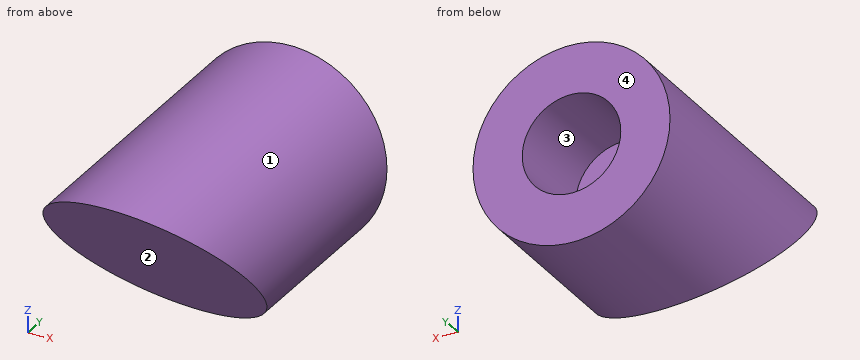
```python
from build123d import *

# Parameters (mm, degrees)
F0_R     = 5
F1_DEPTH = 12.5
F3_W     = 50
F3_H     = 50
F4_DEPTH = 25
F5_R     = 2.5
F6_DEPTH = 5


with BuildPart() as f1:
    # F0 (on Front) → F1 (new body, symmetric)
    with BuildSketch(Plane.XZ):
        Circle(F0_R)
    extrude(amount=F1_DEPTH, both=True)

    # F3 (on face) → F4 (cut)
    with BuildSketch(Plane(origin=(0, 0, 0), x_dir=(-1, 0, 0), z_dir=(0, 0.707107, 0.707107))):
        Rectangle(F3_W, F3_H)
    extrude(amount=-F4_DEPTH, mode=Mode.SUBTRACT)

    # F5 (on face) → F6 (cut)
    with BuildSketch(Plane(origin=(0, 12.5, 0), x_dir=(-1, 0, 0), z_dir=(0, 1, 0))):
        Circle(F5_R)
    extrude(amount=-F6_DEPTH, mode=Mode.SUBTRACT)


solid = f1.part
```
Verification items for the finished model (mm, model axes). Face numbers are marked on the shaded views. Round coordinates to 2 decimals unless told otherwise and drop trailing zeros. Write each loop counter-clockwise with the first axis right and the second up, starting at its lowest first coordinate (ties: lowest second). Pieces come first, ordered by that corner, then holes. Notation, with made-up numbers: (57.25, 54.5) - (113.25, 54.5) arc R19 ccw to (113.25, 61.5) - close; hole circle Ø11 at (83, 58.5). An arc over 180 degrees is marked (long way). Answer as a JSON object with one key per item and string values. Group by question number.
Q1. Section check D-D, the plane y = 10.25. Enter the section's corners in (x, z).
Q2. Section check B-B, the plane x = 0. Enter the section's corners in (y, z), plus the area to 3 significant figures.
Q3. Thickness scan on line 1 (Z direction, x = 0, y = 9.95); line 2 (Z direction, x = -1.75, y = 3.5); line 3 (X direction, y = 2.25, z = 3). Record the ranges inside material, lowest first.
Q4. Mould release check, pull along Z, two halves, no side actions. Record for the marked faces 1, 2, 3 and 4: released by +Z, released by -Z, zero draft, split by the parting line, or undercut.
Q5. Go/stop test with flat-tipped pins: pin 1 Ø4 at (x, z) = (0, 0) entering from +Y; pin 2 Ø2 at (x, z) = (0.5, 0.5) entering from -Y; pin 3 Ø1.5 at (x, y) = (-1.5, 2.5) entering from +Z. Record where each tip stops, or that it passes through.
Q6. Section check C-C, the plane y = -4. Enter the section's corners in (x, z).
Found:
{
 "1": {"outline": "circle Ø10 at (0, 0); hole circle Ø5 at (0, 0)"},
 "2": {"outline": "(-5, 5) - (5, -5) - (12.5, -5) - (12.5, -2.5) - (7.5, -2.5) - (7.5, 2.5) - (12.5, 2.5) - (12.5, 5) - close", "area": "100 mm^2"},
 "3": {"line 1": "z = -5 to -2.5, 2.5 to 5", "line 2": "z = -3.5 to 4.68", "line 3": "x = -4 to 4"},
 "4": {"face 1": "split by the parting line", "face 2": "released by -Z", "face 3": "undercut", "face 4": "zero draft"},
 "5": {"pin 1": "stops at y = 7.5", "pin 2": "stops at y = -1.5", "pin 3": "stops at z = 4.94"},
 "6": {"outline": "(-3, 4) - (3, 4) arc R5 ccw to start"}
}
